Here's how the part is built. I have some questions about the finished solid (model axes, mm). A direction names the side the tool comes from. Give positions to 0.01 mm unless a question says otherwise; leave off trailing zeros. Loops run counter-clockwise (first coordinate to the right, second up) from the corner with the lowest first, then second, coordinate; pieces in that order, holes last. Notation, with made-up numbers: (68, 27.25) - (105, 27.25) arc R23 cw to (105, 36.25) - close; hole circle Ø5 at (-33.75, 70). An arc over 180 degrees is marked (long way). Use a Markdown table: item, result.
from build123d import *

# Parameters (mm, degrees)
ESQUISSE3_W      = 400
ESQUISSE3_H      = 40
EXTRUSION1_DEPTH = 110
ESQUISSE8_W      = 400
ESQUISSE8_H      = 122
EXTRUSION3_DEPTH = 15
ESQUISSE11_W     = 400
ESQUISSE11_H     = 110
EXTRUSION5_DEPTH = 6
ESQUISSE10_R     = 3
EXTRUSION4_DEPTH = 1
ESQUISSE12_R     = 3
EXTRUSION6_DEPTH = 20


with BuildPart() as part:
    # Esquisse3 → Extrusion1 (new body)
    with BuildSketch(Plane.XY):
        with Locations((38, 5)):
            Rectangle(ESQUISSE3_W, ESQUISSE3_H)
    extrude(amount=EXTRUSION1_DEPTH)

    # Esquisse8 → Extrusion3 (add)
    with BuildSketch(Plane(origin=(0, 25, 0), x_dir=(1, 0, 0), z_dir=(0, 1, 0))):
        with Locations((38, -49)):
            Rectangle(ESQUISSE8_W, ESQUISSE8_H)
    extrude(amount=EXTRUSION3_DEPTH)

    # Esquisse11 → Extrusion5 (add)
    with BuildSketch(Plane.XZ.offset(15)):
        with Locations((38, 55)):
            Rectangle(ESQUISSE11_W, ESQUISSE11_H)
    extrude(amount=EXTRUSION5_DEPTH)

    # Esquisse10 → Extrusion4 (cut)
    with BuildSketch(Plane(origin=(0, 0, 0), x_dir=(-1, 0, 0), z_dir=(0, 0, -1))):
        with BuildLine():
            Line((59.5, -8), (59.5, -19))
            ThreePointArc((59.5, -19), (58.914213562, -20.414213562), (57.5, -21))
            Line((57.5, -21), (-68.5, -21))
            ThreePointArc((-68.5, -21), (-69.914213562, -20.414213562), (-70.5, -19))
            Line((-70.5, -19), (-70.5, -8))
            ThreePointArc((-70.5, -8), (-71.085786438, -6.585786438), (-72.5, -6))
            Line((-72.5, -6), (-83, -6))
            ThreePointArc((-83, -6), (-95.5, 6.5), (-83, 19))
            Line((-83, 19), (70.25, 19))
            ThreePointArc((70.25, 19), (82.75, 6.5), (70.25, -6))
            Line((70.25, -6), (61.5, -6))
            ThreePointArc((61.5, -6), (60.085786438, -6.585786438), (59.5, -8))
        make_face()
        with Locations((-86.5, 6.5)):
            Circle(ESQUISSE10_R, mode=Mode.SUBTRACT)
        with Locations((-20.5, 6.5)):
            Circle(ESQUISSE10_R, mode=Mode.SUBTRACT)
        with Locations((72.75, 6.5)):
            Circle(ESQUISSE10_R, mode=Mode.SUBTRACT)
        with BuildLine():
            Line((-31.5, -3), (-61.5, -3))
            ThreePointArc((-61.5, -3), (-62.207106781, -2.707106781), (-62.5, -2))
            Line((-62.5, -2), (-62.5, 12))
            ThreePointArc((-62.5, 12), (-62.207106781, 12.707106781), (-61.5, 13))
            Line((-61.5, 13), (-31.5, 13))
            ThreePointArc((-31.5, 13), (-30.792893219, 12.707106781), (-30.5, 12))
            Line((-30.5, 12), (-30.5, -2))
            ThreePointArc((-30.5, -2), (-30.792893219, -2.707106781), (-31.5, -3))
        make_face(mode=Mode.SUBTRACT)
        with BuildLine():
            Line((51.75, 0), (12.75, 0))
            ThreePointArc((12.75, 0), (12.042893219, 0.292893219), (11.75, 1))
            Line((11.75, 1), (11.75, 11))
            ThreePointArc((11.75, 11), (12.042893219, 11.707106781), (12.75, 12))
            Line((12.75, 12), (51.75, 12))
            ThreePointArc((51.75, 12), (52.457106781, 11.707106781), (52.75, 11))
            Line((52.75, 11), (52.75, 1))
            ThreePointArc((52.75, 1), (52.457106781, 0.292893219), (51.75, 0))
        make_face(mode=Mode.SUBTRACT)
    extrude(amount=-EXTRUSION4_DEPTH, mode=Mode.SUBTRACT)

    # Esquisse12 → Extrusion6 (cut)
    with BuildSketch(Plane(origin=(0, 0, 0), x_dir=(-1, 0, 0), z_dir=(0, 0, -1))):
        with Locations((-86.5, 6.5)):
            Circle(ESQUISSE12_R)
        with Locations((-20.5, 6.5)):
            Circle(ESQUISSE12_R)
        with Locations((72.75, 6.5)):
            Circle(ESQUISSE12_R)
        with BuildLine():
            Line((-30.5, -2), (-30.5, 12))
            ThreePointArc((-30.5, 12), (-30.792893219, 12.707106781), (-31.5, 13))
            Line((-31.5, 13), (-61.5, 13))
            ThreePointArc((-61.5, 13), (-62.207106781, 12.707106781), (-62.5, 12))
            Line((-62.5, 12), (-62.5, -2))
            ThreePointArc((-62.5, -2), (-62.207106781, -2.707106781), (-61.5, -3))
            Line((-61.5, -3), (-31.5, -3))
            ThreePointArc((-31.5, -3), (-30.792893219, -2.707106781), (-30.5, -2))
        make_face()
        with BuildLine():
            Line((52.75, 1), (52.75, 11))
            ThreePointArc((52.75, 11), (52.457106781, 11.707106781), (51.75, 12))
            Line((51.75, 12), (12.75, 12))
            ThreePointArc((12.75, 12), (12.042893219, 11.707106781), (11.75, 11))
            Line((11.75, 11), (11.75, 1))
            ThreePointArc((11.75, 1), (12.042893219, 0.292893219), (12.75, 0))
            Line((12.75, 0), (51.75, 0))
            ThreePointArc((51.75, 0), (52.457106781, 0.292893219), (52.75, 1))
        make_face()
    extrude(amount=-EXTRUSION6_DEPTH, mode=Mode.SUBTRACT)


solid = part.part
(1) Suppose I cut it at B-B on x = 45.5. Write out the boundary of the cut face in (y, z).
A:
| item | result |
|---|---|
| outline | (-21, 1) - (-3, 1) - (-3, 20) - (13, 20) - (13, 1) - (19, 1) - (19, 0) - (25, 0) - (25, -12) - (40, -12) - (40, 110) - (-21, 110) - close |
(2) Suppose I cut it at A-A on z = 16. Write out the boundary of the cut face in (x, y).
A:
| item | result |
|---|---|
| outline | (-162, -21) - (238, -21) - (238, 40) - (-162, 40) - close; hole circle Ø6 at (-72.75, 6.5); hole (-52.75, 1) arc R1 ccw to (-51.75, 0) - (-12.75, 0) arc R1 ccw to (-11.75, 1) - (-11.75, 11) arc R1 ccw to (-12.75, 12) - (-51.75, 12) arc R1 ccw to (-52.75, 11) - close; hole circle Ø6 at (20.5, 6.5); hole (30.5, -2) arc R1 ccw to (31.5, -3) - (61.5, -3) arc R1 ccw to (62.5, -2) - (62.5, 12) arc R1 ccw to (61.5, 13) - (31.5, 13) arc R1 ccw to (30.5, 12) - close; hole circle Ø6 at (86.5, 6.5) |
(3) Suppose I cut it at C-C on x = -29.5. Write out the boundary of the cut face in (y, z), plus the area to 3 significant figures.
A:
| item | result |
|---|---|
| outline | (-21, 1) - (0, 1) - (0, 20) - (12, 20) - (12, 1) - (19, 1) - (19, 0) - (25, 0) - (25, -12) - (40, -12) - (40, 110) - (-21, 110) - close |
| area | 6,620 mm2 |
(4) If I drill on line 1 (X direction, y = 6, z = 7); line 2 (Y direction, x = -73, z = 8); line 3 (Z direction, x = -138, y = -15), over which ranges is the centre line in solid material (lowest first)?
A:
| item | result |
|---|---|
| line 1 | -162 to -75.71, -69.79 to -52.75, -11.75 to 17.54, 23.46 to 30.5, 62.5 to 83.54, 89.46 to 238 |
| line 2 | -21 to 3.51, 9.49 to 40 |
| line 3 | 0 to 110 |
(5) Will these pins go through, and if not, where does the flat tip stop? pin 1 (8 mm diameter, centred on x = 49, y = 6, fed in from -Z); pin 2 (1 mm diameter, centred on x = -121, y = 17, fed in from -Z); pin 3 (2 mm diameter, centred on x = -52, y = -8.5, fed in from -Z).
A:
| item | result |
|---|---|
| pin 1 | z = 20 |
| pin 2 | z = 0 |
| pin 3 | z = 1 |
(6) Suppose I cut it at D-D on x = 181. Write out the boundary of the cut face in (y, z), plus the area to 3 significant figures.
A:
| item | result |
|---|---|
| outline | (-21, 0) - (25, 0) - (25, -12) - (40, -12) - (40, 110) - (-21, 110) - close |
| area | 6,890 mm2 |
(7) On a 3-axis mill with a long thin cutter (end or side, diameter ignored), from which of +Z, -Z, +X, -X, +Y, -Y can I reach the whole of each face in a straight line? I mean faces 1 (the face through (-52.75, 6, 10)), 2 (the face through (35, 23, 0)), 3 (the face through (35, 10, 110)). Say none if no direction works.
A:
| item | result |
|---|---|
| face 1 | -Z |
| face 2 | -Z, +X, -X, -Y |
| face 3 | +Z, +X, -X, +Y, -Y |
(8) We'd pull the mould along X, two halves only. Please class faces 4 (the face through (95.497, 6.225, 0.493)), 5 (the face through (35, -21, 56)), 6 (the face through (-32, 6, 20)): pulls with the +X half, pulls with the -X half, needs draft (parallel to the pull), parting line crosses it, or undercut.
A:
| item | result |
|---|---|
| face 4 | undercut |
| face 5 | needs draft |
| face 6 | undercut |
